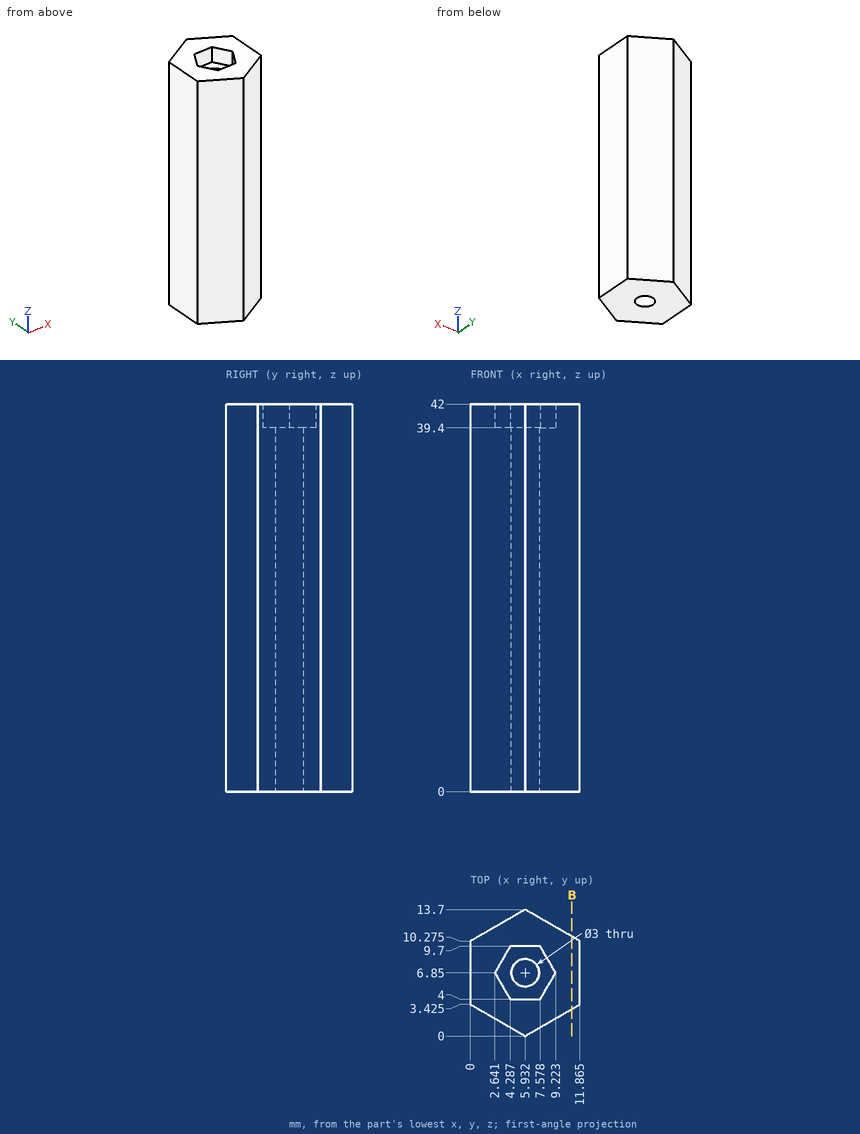
Verification items for this drawing (mm, ordinates from the low corner). Coordinates: 2 decimals unless noted, no trailing zeros. Write each loop counter-clockwise with the first axis right and the second up, starting at its lowest first coordinate (ties: lowest second). Pieces come first, ordered by that corner, then holes. Notation, with made-up numbers: M -32,33 L -24,33 A17 cw -24,52 Z; hole C 63.5,24.25 d7. An arc over 180 degrees is marked long. Answer as a JSON object with one key per item and string values. Group by question number.
(1) Material ranges on line 1 (X direction, y = 6.85, z = 26) (1 decimal); line 2 (Y direction, x = 4.75, z = 2) (1 decimal); line 3 (Y direction, x = 6.5, z = 17), recorded low to high.
(2) Cross-section at B-B, the plane x = 11. Record the cut outline in (y, z) (1 decimal), and give its area (3 significant figures).
(3) Gauge pin test, flat ends, axial feed: pin 1 (1 mm diameter, centred on x = 1.5, y = 3, fed in from -Z); pin 2 (1 mm diameter, centred on x = 10.5, z = 35.5, fed in from -Y); pin 3 (1.3 mm diameter, centred on x = 5, z = 40.5, fed in from -Y); pin 4 (5 mm diameter, centred on x = 5.93, y = 6.85, fed in from +Z). Record the tip position at first contact, or that the pin passes through.
Reply:
{
 "1": {"line 1": "0 to 4.4, 7.4 to 11.9", "line 2": "0.7 to 5.9, 7.8 to 13", "line 3": "0.33 to 5.46, 8.24 to 13.37"},
 "2": {"outline": "M 2.9,0 L 10.8,0 L 10.8,42 L 2.9,42 Z", "area": "330 mm²"},
 "3": {"pin 1": "z = 0", "pin 2": "y = 2.35", "pin 3": "y = 0.16", "pin 4": "z = 39.4"}
}
